For this review, take the finished solid that the model builds, in its own axes (mm). A direction names the side the tool comes from. Give positions to 0.01 mm unless a question says otherwise; leave off trailing zeros. Order: outer loops, then holes, each group sorted by start corner. A loop starts at its lowest first (then second) coordinate and runs counter-clockwise, first axis right, second up.
Item 1: Consider section A-A (z = 10). Give the boundary of the cut face in (x, y), plus the area to 3 significant figures.
Item 2: Consider section B-B (y = -22.5). Give the boundary of the cut face in (x, z).
Item 3: Machinability: for faces 4 (the cylindrical face through (-2, 1.9, 4)), 5 (the flat face through (0, 3, 6)), 6 (the flat face through (-2.2, -2.2, 2)), which of the approach directions +Z, -Z, +X, -X, +Y, -Y give a long, thin tool a straight path to every point of the face, cutting with its end or side? Answer none if there is none.
Item 4: The part is to be moulded in two halves that separate along X. For faces 1 (the flat face through (1, 12, 0)), 2 (the cylindrical face through (-16.128, 70.296, 9.86)), 3 (the flat face through (39, -22, 3)), say which applies: released by +X, released by -X, zero draft, split by the parting line, or undercut.
Item 5: For probe 1 along Y at (x, z) = (0, 0.95); probe 2 along X at (y, z) = (-40, 8.5); probe 3 along Y at (x, z) = (0, 12.25), list the stretches that pass through material, from the lowest coordinate up.
Item 6: For P1, Ø5, axis at x = -50.5, y = -21.5, coming from the +Z side; P2, Ø5, axis at y = -27.5, z = 12, coming from the +X side; P3, Ø2.5, axis at x = -6.06, y = 3.5, coming from the -Z side; P4, Ø10, axis at x = 19, z = 10.5, coming from the -Y side, all flat-tipped, find the tip position at first contact; note any pin that passes through.
Item 7: Consider section D-D (y = 22). Give the boundary of the cut face in (x, z), plus the area to 3 significant figures.
Item 8: Consider section C-C (x = 49.5). Give the boundary of the cut face in (y, z).
```python
from build123d import *

# Parameters (mm, degrees)
SKETCH_1_R          = 17.5
SKETCH_1_R_2        = 1
SKETCH_1_R_3        = 2.759956758
EXTRUDE_1_DEPTH     = 6
SKETCH_2_R          = 5
CUT_EXTRUDE_1_DEPTH = 2
SKETCH_4_R          = 30
EXTRUDE_2_DEPTH     = 20
SKETCH_5_R          = 27.5
CUT_EXTRUDE_2_DEPTH = 17


with BuildPart() as part:
    # 草图1 → 凸台-拉伸1 (new body)
    with BuildSketch(Plane.XY):
        Circle(SKETCH_1_R)
        with Locations((7, 0)):
            Circle(SKETCH_1_R_2, mode=Mode.SUBTRACT)
        with Locations((6.062177826, -3.5)):
            Circle(SKETCH_1_R_2, mode=Mode.SUBTRACT)
        with Locations((3.5, -6.062177826)):
            Circle(SKETCH_1_R_2, mode=Mode.SUBTRACT)
        with Locations((0, -7)):
            Circle(SKETCH_1_R_2, mode=Mode.SUBTRACT)
        with Locations((-3.5, -6.062177826)):
            Circle(SKETCH_1_R_2, mode=Mode.SUBTRACT)
        with Locations((-6.062177826, -3.5)):
            Circle(SKETCH_1_R_2, mode=Mode.SUBTRACT)
        with Locations((-7, 0)):
            Circle(SKETCH_1_R_2, mode=Mode.SUBTRACT)
        with Locations((-6.062177826, 3.5)):
            Circle(SKETCH_1_R_2, mode=Mode.SUBTRACT)
        with Locations((-3.5, 6.062177826)):
            Circle(SKETCH_1_R_2, mode=Mode.SUBTRACT)
        with Locations((0, 7)):
            Circle(SKETCH_1_R_2, mode=Mode.SUBTRACT)
        with Locations((3.5, 6.062177826)):
            Circle(SKETCH_1_R_2, mode=Mode.SUBTRACT)
        with Locations((6.062177826, 3.5)):
            Circle(SKETCH_1_R_2, mode=Mode.SUBTRACT)
        Circle(SKETCH_1_R_3, mode=Mode.SUBTRACT)
    extrude(amount=EXTRUDE_1_DEPTH)

    # 草图2 → 切除-拉伸1 (cut)
    with BuildSketch(Plane(origin=(0, 0, 0), x_dir=(-1, 0, 0), z_dir=(0, 0, -1))):
        Circle(SKETCH_2_R)
    extrude(amount=-CUT_EXTRUDE_1_DEPTH, mode=Mode.SUBTRACT)

    # 草图4 → 凸台-拉伸2 (add)
    with BuildSketch(Plane(origin=(0, 0, 0), x_dir=(-1, 0, 0), z_dir=(0, 0, -1))):
        with Locations((0, 45)):
            Circle(SKETCH_4_R)
        with Locations((38.97114317, -22.5)):
            Circle(SKETCH_4_R)
        with Locations((-38.97114317, -22.5)):
            Circle(SKETCH_4_R)
    extrude(amount=-EXTRUDE_2_DEPTH)

    # 草图5 → 切除-拉伸2 (cut)
    with BuildSketch(Plane.XY.offset(20)):
        with Locations((0, 45)):
            Circle(SKETCH_5_R)
        with Locations((38.97114317, -22.5)):
            Circle(SKETCH_5_R)
        with Locations((-38.97114317, -22.5)):
            Circle(SKETCH_5_R)
    extrude(amount=-CUT_EXTRUDE_2_DEPTH, mode=Mode.SUBTRACT)


solid = part.part
```
Resolved:
1. outline: circle Ø60 at (-38.97, -22.5); circle Ø60 at (0, 45); circle Ø60 at (38.97, -22.5); hole circle Ø55 at (-38.97, -22.5); hole circle Ø55 at (0, 45); hole circle Ø55 at (38.97, -22.5)
1. area: 1,350 mm2
2. outline: (-68.97, 0) - (-8.97, 0) - (-8.97, 20) - (-11.47, 20) - (-11.47, 3) - (-66.47, 3) - (-66.47, 20) - (-68.97, 20) - close; (8.97, 0) - (68.97, 0) - (68.97, 20) - (66.47, 20) - (66.47, 3) - (11.47, 3) - (11.47, 20) - (8.97, 20) - close
3. face 4: +Z, -Z
3. face 5: +Z
3. face 6: -Z
4. face 1: zero draft
4. face 2: split by the parting line
4. face 3: undercut
5. probe 1: y = -17.5 to -8, -6 to -5, 5 to 6, 8 to 75
5. probe 2: x = -63.34 to -60.18, -17.76 to -14.6, 14.6 to 17.76, 60.18 to 63.34
5. probe 3: y = 15 to 17.5, 72.5 to 75
6. P1: stops at z = 3
6. P2: stops at x = 68.87
6. P3: stops at z = 0
6. P4: stops at y = -48.5
7. outline: (-19.26, 0) - (19.26, 0) - (19.26, 20) - (15.07, 20) - (15.07, 3) - (-15.07, 3) - (-15.07, 20) - (-19.26, 20) - close
7. area: 258 mm2
8. outline: (-50.59, 0) - (5.59, 0) - (5.59, 20) - (2.9, 20) - (2.9, 3) - (-47.9, 3) - (-47.9, 20) - (-50.59, 20) - close
